Here's how the part is built. I have some questions about the finished solid (model axes, mm). A direction names the side the tool comes from. Coordinates: 2 decimals unless noted, no trailing zeros. Write each loop counter-clockwise with the first axis right and the second up, starting at its lowest first coordinate (ties: lowest second). Pieces come first, ordered by that corner, then holes.
```python
from build123d import *

# Parameters (mm, degrees)
SKETCH1_R                       = 1.55
SKETCH1_R_2                     = 2.45
BOSS_EXTRUDE1_DEPTH             = 10
SKETCH2_W                       = 9.45
SKETCH2_H                       = 1.5
CUT_EXTRUDE1_DEPTH              = 25.542893997
BOSS_EXTRUDE3_DEPTH             = 10
BOSS_EXTRUDE4_DEPTH             = 15
F_3_0MM_CLEARANCE_DOWEL_HOLE1_D = 3.108
FILLET1_R                       = 5


with BuildPart() as part:
    # Sketch1 → Boss-Extrude1 (new body)
    with BuildSketch(Plane(origin=(0, 0, 0), x_dir=(1, 0, 0), z_dir=(0, 1, 0))):
        with BuildLine():
            Line((11.25, 2.165063509), (-2.121223771, 9.884943153))
            ThreePointArc((-2.121223771, 9.884943153), (-7.442989886, 11.219511103), (-12.667897108, 9.545411133))
            Line((-12.667897108, 9.545411133), (-15.191606303, 7.863082307))
            ThreePointArc((-15.191606303, 7.863082307), (-19.4, 0), (-15.191606303, -7.863082307))
            Line((-15.191606303, -7.863082307), (-12.667897108, -9.545411133))
            ThreePointArc((-12.667897108, -9.545411133), (-7.442989886, -11.219511103), (-2.121223771, -9.884943153))
            Line((-2.121223771, -9.884943153), (11.25, -2.165063509))
            ThreePointArc((11.25, -2.165063509), (12.5, 0), (11.25, 2.165063509))
        make_face()
        with Locations(Location((7.5, 0, 0), (0, 0, 270))):
            Circle(SKETCH1_R, mode=Mode.SUBTRACT)
        with Locations(Location((-3.75, 6.495190528, 0), (0, 0, 270))):
            Circle(SKETCH1_R, mode=Mode.SUBTRACT)
        with Locations(Location((-9.95, 0, 0), (0, 0, 270))):
            Circle(SKETCH1_R_2, mode=Mode.SUBTRACT)
    extrude(amount=BOSS_EXTRUDE1_DEPTH)

    # Sketch2 → Cut-Extrude1 (cut, through all)
    with BuildSketch(Plane(origin=(0, 10, 0), x_dir=(1, 0, 0), z_dir=(0, 1, 0))):
        with Locations((-14.675, 0)):
            Rectangle(SKETCH2_W, SKETCH2_H)
    extrude(amount=-CUT_EXTRUDE1_DEPTH, mode=Mode.SUBTRACT)

    # Sketch3 → Boss-Extrude3 (add)
    with BuildSketch(Plane.XZ):
        with BuildLine():
            Line((-35.868683143, 22.59247598), (-22.285990587, -0.93343763))
            Line((-22.285990587, -0.93343763), (-19.370191081, 0.75))
            ThreePointArc((-19.370191081, 0.75), (-18.098070975, 4.786589536), (-15.191606303, 7.863082307))
            Line((-15.191606303, 7.863082307), (-12.667897108, 9.545411133))
            Line((-12.667897108, 9.545411133), (-31.538556124, 25.09247598))
            Line((-31.538556124, 25.09247598), (-35.868683143, 22.59247598))
        make_face()
    extrude(amount=-BOSS_EXTRUDE3_DEPTH)

    # Sketch4 → Boss-Extrude4 (add)
    with BuildSketch(Plane(origin=(0, 10, 0), x_dir=(1, 0, 0), z_dir=(0, 1, 0))):
        Polygon((-35.868683143, -22.59247598), (-25.868683143, -5.271967904), (-21.538556124, -7.771967904), (-31.538556124, -25.09247598), align=None)
    extrude(amount=BOSS_EXTRUDE4_DEPTH)

    # Ø3.0mm Clearance Dowel Hole1 (through all)
    with Locations(Plane(origin=(-12.788556272, 0, -7.383476406), x_dir=(0.5000000000000013, 0, -0.8660254037844379), z_dir=(0.8660254037844379, 0, 0.5000000000000013))):
        with Locations((-32.499999704, 17.5), (-22.499999704, 17.5)):
            Hole(F_3_0MM_CLEARANCE_DOWEL_HOLE1_D / 2)

    # Fillet1
    fillet1_edges = [part.edges().sort_by_distance(p)[0] for p in [
        (-12.667897108, 5, 9.545411133),
    ]]
    fillet(fillet1_edges, radius=FILLET1_R)


solid = part.part
```
1) I need wall thicknesses on probe 1 along Y at (x, z) = (-25, 16.5); probe 2 along Z at (x, y) = (-9.95, 6.25); probe 3 along Z at (x, y) = (-12, 2.25). Which ranges of each line are inside material? Lowest first, please.
Values follow:
probe 1: y = 0 to 10
probe 2: z = -10.82 to -2.45, 2.45 to 10.82
probe 3: z = -9.95 to -1.34, 1.34 to 10.43
2) Imagine slicing it at D-D on x = -18.5. Please give me the cut outline in (y, z), then the cut area to 3 significant figures.
Values follow:
outline: (0, -4.02) - (10, -4.02) - (10, -0.75) - (0, -0.75) - close; (0, 0.75) - (10, 0.75) - (10, 14.35) - (0, 14.35) - close
area: 169 mm2
3) We'd pull the mould along Z, two halves only. Please class faces 1 (the face through (-16, 5, 0.75)), 2 (the face through (-33.67, 12.32, 23.86)), 3 (the face through (-13.912, 4.93, -8.716)): pulls with the +Z half, pulls with the -Z half, needs draft (parallel to the pull), parting line crosses it, or undercut.
Values follow:
face 1: undercut
face 2: pulls with the +Z half
face 3: pulls with the -Z half
4) Imagine slicing it at A-A on z = 0. Please give me the cut outline in (x, y).
Values follow:
outline: (-22.82, 0) - (-20.67, 0) - (-20.67, 10) - (-22.82, 10) - close; (-7.5, 0) - (5.95, 0) - (5.95, 10) - (-7.5, 10) - close; (9.05, 0) - (12.5, 0) - (12.5, 10) - (9.05, 10) - close
5) Will these pins go through, and if not, where does the flat tip stop? pin 1 (3 mm diameter, centred on x = 7.5, z = 0, fed in from -Y); pin 2 (2 mm diameter, centred on y = 20.5, z = 6.5, fed in from -X); pin 3 (5 mm diameter, centred on x = -15.5, y = 10, fed in from -Z); pin 4 (8 mm diameter, centred on x = -17.5, y = 4.5, fed in from -Z).
Values follow:
pin 1: passes through
pin 2: stops at x = -27.16
pin 3: stops at z = -9.32
pin 4: stops at z = -8.99
6) Imagine slicing it at B-B on x = -11. Please give me the cut outline in (y, z).
Values follow:
outline: (0, -10.44) - (10, -10.44) - (10, -2.21) - (0, -2.21) - close; (0, 2.21) - (10, 2.21) - (10, 10.52) - (0, 10.52) - close
7) On a 3-axis mill with a long thin cutter (end or side, diameter ignored), from which of +Z, -Z, +X, -X, +Y, -Y can I reach the whole of each face in a straight line? I mean faces 4 (the face through (-26.47, 17.4, 16.31)), 5 (the face through (-7.502, 4.93, 0.097)), 6 (the face through (-23.734, 17.395, 6.504)). Say none if no direction works.
Values follow:
face 4: +Z, +X, +Y
face 5: +Y, -Y
face 6: -Z, +X, +Y
8) Imagine slicing it at C-C on y = 11. Please give me the cut outline in (x, z), then the cut area to 3 significant figures.
Values follow:
outline: (-35.87, 22.59) - (-25.87, 5.27) - (-21.54, 7.77) - (-31.54, 25.09) - close
area: 100 mm2
